Input: part model. Units: mm. Frame: model coordinates. A direction names the side the tool comes from. Coordinates: 2 decimals unless noted, no trailing zeros. Loops run counter-clockwise (first coordinate to the right, second up) from the corner with the lowest first, then second, coordinate; pieces in that order, holes last.
```python
from build123d import *

# Parameters (mm, degrees)
SKETCH_2_R        = 3
EXTRUDE_1_DEPTH   = 5
EXTRUDE_1_2_DEPTH = 5
SKETCH_2_3_R      = 40
SKETCH_2_3_R_2    = 6
SKETCH_2_3_R_3    = 12.5
EXTRUDE_2_DEPTH   = 10


with BuildPart() as part:
    # Sketch 2 → Extrude 1 (new body)
    with BuildSketch(Plane.XY):
        with BuildLine():
            ThreePointArc((63, -20), (83, 0), (63, 20))
            Line((63, 20), (40.987803064, 20))
            ThreePointArc((40.987803064, 20), (35.725454948, 21.215395589), (31.52907928, 24.615384615))
            ThreePointArc((31.52907928, 24.615384615), (40, 0), (31.52907928, -24.615384615))
            ThreePointArc((31.52907928, -24.615384615), (35.725454948, -21.215395589), (40.987803064, -20))
            Line((40.987803064, -20), (63, -20))
        make_face()
        with Locations((69, -10.392304845)):
            Circle(SKETCH_2_R, mode=Mode.SUBTRACT)
        with Locations((51, 0)):
            Circle(SKETCH_2_R, mode=Mode.SUBTRACT)
        with Locations((69, 10.392304845)):
            Circle(SKETCH_2_R, mode=Mode.SUBTRACT)
    extrude(amount=EXTRUDE_1_DEPTH)



with BuildPart() as body_2:
    # Sketch 2 → Extrude 1 2 (new body)
    with BuildSketch(Plane.XY):
        with BuildLine():
            ThreePointArc((-17.959183673, -35.741680455), (-39.592499474, -5.695084317), (-27.304983614, 29.230769231))
            ThreePointArc((-27.304983614, 29.230769231), (-31.093682384, 26.836873887), (-35.496478699, 26))
            Line((-35.496478699, 26), (-92, 26))
            ThreePointArc((-92, 26), (-99.071067812, 28.928932188), (-102, 36))
            Line((-102, 36), (-102, -87.567117116))
            ThreePointArc((-102, -87.567117116), (-74.443658232, -38.199276638), (-17.959183673, -35.741680455))
        make_face()
        with BuildLine():
            ThreePointArc((-99, 0), (-96.656854249, 5.656854249), (-91, 8))
            Line((-91, 8), (-52.617915552, 8))
            ThreePointArc((-52.617915552, 8), (-42.630507284, -1.498326705), (-51.615832348, -11.949664781))
            ThreePointArc((-51.615832348, -11.949664781), (-69.852655287, -16.099360648), (-86.523809524, -24.577232027))
            ThreePointArc((-86.523809524, -24.577232027), (-94.754362542, -25.011048058), (-99, -17.946717807))
            Line((-99, -17.946717807), (-99, 0))
        make_face(mode=Mode.SUBTRACT)
    extrude(amount=EXTRUDE_1_2_DEPTH)


with BuildPart() as part_1:
    add(part.part)

    add(body_2.part)  # Extrude 2 merges body 2
    # Sketch 2_3 → Extrude 2 (add)
    # profile 1 of 2: a face of its own
    with BuildSketch(Plane.XY):
        with BuildLine():
            Line((-118, 58), (-118, -112))
            ThreePointArc((-118, -112), (-106.686291501, -107.313708499), (-102, -96))
            Line((-102, -96), (-102, 42))
            ThreePointArc((-102, 42), (-106.686291501, 53.313708499), (-118, 58))
        make_face()
    # profile 2 of 2: a face of its own
    with BuildSketch(Plane.XY):
        with Locations(Location((0, 0, 0), (0, 0, 133.0490798))):
            Circle(SKETCH_2_3_R)
        with Locations((-18.384776311, 18.384776311)):
            Circle(SKETCH_2_3_R_2, mode=Mode.SUBTRACT)
        with Locations((-26, 0)):
            Circle(SKETCH_2_3_R_2, mode=Mode.SUBTRACT)
        with Locations((-18.384776311, -18.384776311)):
            Circle(SKETCH_2_3_R_2, mode=Mode.SUBTRACT)
        with Locations((0, -26)):
            Circle(SKETCH_2_3_R_2, mode=Mode.SUBTRACT)
        with Locations((18.384776311, -18.384776311)):
            Circle(SKETCH_2_3_R_2, mode=Mode.SUBTRACT)
        with Locations((26, 0)):
            Circle(SKETCH_2_3_R_2, mode=Mode.SUBTRACT)
        with Locations((18.384776311, 18.384776311)):
            Circle(SKETCH_2_3_R_2, mode=Mode.SUBTRACT)
        with Locations((0, 26)):
            Circle(SKETCH_2_3_R_2, mode=Mode.SUBTRACT)
        Circle(SKETCH_2_3_R_3, mode=Mode.SUBTRACT)
    extrude(amount=EXTRUDE_2_DEPTH)


solid = part_1.part
```
Item 1: Mould query, pull axis X, two halves, no side actions, for faces 1 (the face through (-98.99, 28.85, 2.46)), 2 (the face through (-102, -28, 7)), 3 (the face through (52, 20, 2)), 4 (the face through (-118, -26, 5)). Classes: +X half, -X half, draft (parallel to the pull), parting line (faces both ways), or undercut.
Result:
face 1: undercut
face 2: undercut
face 3: draft
face 4: -X half
Item 2: Contact query for flat-ended pins moving along their axis: P1, Ø9.5, axis at x = -18.38, y = -18.38, coming from the -Z side; P2, Ø1.5, axis at x = 54.5, z = 3, coming from the +Y side; P3, Ø5, axis at x = -67.5, z = 2, coming from the +Y side; P4, Ø15, axis at x = 55.5, y = -8.5, coming from the +Z side. Output: stop coordinate, or through.
Result:
P1: passes through
P2: stops at y = 20
P3: stops at y = 26
P4: stops at z = 5
Item 3: Line query: L1, parallel to Y at x = 0, z = 2.5; L2, parallel to X at y = -27, z = 6.5; L3, parallel to X at y = -17, z = 6.25. Output: solid intervals per line, ascending.
Result:
L1: y = -40 to -32, -20 to -12.5, 12.5 to 20, 32 to 40
L2: x = -118 to -102, -29.51 to -5.92, 5.92 to 29.51
L3: x = -118 to -102, -36.21 to -24.22, -12.55 to 12.55, 24.22 to 36.21
Item 4: Reachability of faces 5 (the face through (-106.563, 53.189, 4.93)), 6 (the face through (-96.719, 5.594, 2.465)) from +Z, -Z, +X, -X, +Y, -Y: full face, straight path, thin tool, end or side. Return the list, or none.
Result:
face 5: +Z, -Z, +X, +Y
face 6: +Z, -Z
Item 5: Section query D-D (x = -95). Output: boundary loops of the cut face in (y, z), then the cut area to 3 significant figures.
Result:
outline: (-59.94, 0) - (-24.87, 0) - (-24.87, 5) - (-59.94, 5) - close; (6.93, 0) - (26.46, 0) - (26.46, 5) - (6.93, 5) - close
area: 273 mm2
Item 6: Section query A-A (x = 0). Output: boundary loops of the cut face in (y, z).
Result:
outline: (-40, 0) - (-32, 0) - (-32, 10) - (-40, 10) - close; (-20, 0) - (-12.5, 0) - (-12.5, 10) - (-20, 10) - close; (12.5, 0) - (20, 0) - (20, 10) - (12.5, 10) - close; (32, 0) - (40, 0) - (40, 10) - (32, 10) - close
Item 7: Section query C-C (x = 51). Output: boundary loops of the cut face in (y, z), then the cut area to 3 significant figures.
Result:
outline: (-20, 0) - (-3, 0) - (-3, 5) - (-20, 5) - close; (3, 0) - (20, 0) - (20, 5) - (3, 5) - close
area: 170 mm2
Item 8: Section query B-B (z = 7.25). Count the separate pieces of the cut face and the enclosed holes in it, then the cut area to 3 significant figures.
Result:
separate pieces: 2
enclosed holes: 9
area: 6,240 mm2
